Can you work these out from the model? Positions are in its coordinate system, mm. Round coordinates to 2 decimals unless told otherwise and drop trailing zeros. Write each loop counter-clockwise with the first axis right and the second up, starting at its lowest first coordinate (ties: lowest second). Pieces come first, ordered by that corner, then holes.
Q1. If we section it at B-B (z = 70.5): Please give me the cut outline in (x, y), plus the area to 3 significant figures.
Q2. If we section it at A-A (x = 3): Please give me the cut outline in (y, z).
Q3. I'm going to push flat-ended pins straight in: pin 1 Ø2 at (x, y) = (8, -104) entering from -Z; pin 2 Ø10.5 at (x, z) = (0.47, 0) entering from +Y. Where does each tip first touch, or does it pass through?
Q4. If we section it at C-C (y = -30): Please give me the cut outline in (x, z).
Q5. Please list where these lines run through material, in increasing order: line 1 along Z through (x, y) = (4.5, -83); line 2 along X through (y, z) = (-11, 68); line 3 along Z through (x, y) = (-2.5, -14).
Q6. We'd pull the mould along X, two halves only. Please class faces 1 (the cylindrical face through (0.191, -62.611, -12.697)), 2 (the cylindrical face through (3.66, -62.61, -5.01)), 3 (the flat face through (-12.23, -63, 34)): +X half, -X half, draft (parallel to the pull), parting line (faces both ways), or undercut.
Q7. If we section it at D-D (x = -8.25): Please give me the cut outline in (y, z).
from build123d import *

# Parameters (mm, degrees)
F0_R     = 5.827895928
F1_DEPTH = 127


with BuildPart() as f1:
    # F0 (on Front) → F1 (new body)
    with BuildSketch(Plane.XZ):
        with BuildLine():
            ThreePointArc((-5.4695284326, 0), (0.470370132, 5.9398985646), (6.4102686966, 0))
            Line((6.4102686966, 0), (13.170370132, 0))
            Line((13.170370132, 0), (13.170370132, 67.8557001903))
            ThreePointArc((13.170370132, 67.8557001903), (0.4559546677, 80.5557083531), (-12.229629868, 67.8269019314))
            Line((-12.229629868, 67.8269019314), (-12.229629868, 0))
            Line((-12.229629868, 0), (-5.4695284326, 0))
        make_face()
        with Locations((0.4703538064, 67.8557001903)):
            Circle(F0_R, mode=Mode.SUBTRACT)
        with BuildLine():
            Line((13.170370132, 0), (6.4102686966, 0))
            ThreePointArc((6.4102686966, 0), (0.470370132, -5.9398985646), (-5.4695284326, 0))
            Line((-5.4695284326, 0), (-12.229629868, 0))
            ThreePointArc((-12.229629868, 0), (0.470370132, -12.7), (13.170370132, 0))
        make_face()
    extrude(amount=F1_DEPTH)


solid = f1.part
A:
1. outline: (-11.95, -127) - (-4.72, -127) - (-4.72, 0) - (-11.95, 0) - close; (5.66, -127) - (12.89, -127) - (12.89, 0) - (5.66, 0) - close
1. area: 1,840 mm2
2. outline: (-127, -12.45) - (0, -12.45) - (0, -5.37) - (-127, -5.37) - close; (-127, 5.37) - (0, 5.37) - (0, 62.61) - (-127, 62.61) - close; (-127, 73.11) - (0, 73.11) - (0, 80.3) - (-127, 80.3) - close
3. pin 1: stops at z = -10.89
3. pin 2: passes through
4. outline: (-12.23, 0) arc R12.7 ccw to (13.17, 0) - (13.17, 67.86) arc R12.7 ccw to (-12.23, 67.83) - close; hole circle Ø11.88 at (0.47, 0); hole circle Ø11.66 at (0.47, 67.86)
5. line 1: z = -12.04 to -4.36, 4.36 to 63.65, 72.07 to 79.9
5. line 2: x = -12.23 to -5.36, 6.3 to 13.17
5. line 3: z = -12.35 to -5.14, 5.14 to 62.84, 72.87 to 80.2
6. face 1: parting line
6. face 2: undercut
6. face 3: -X half
7. outline: (-127, -9.23) - (0, -9.23) - (0, 77.09) - (-127, 77.09) - close
